Autodesk Inventor part; units mm, degrees
ref_plane "YZ Plane" through (0, 0, 0) normal (1, 0, 0) x (0, 1, 0)
ref_plane "XZ Plane" through (0, 0, 0) normal (0, 1, 0) x (-1, 0, 0)
ref_plane "XY Plane" through (0, 0, 0) normal (0, 0, 1) x (1, 0, 0)
sketch "Sketch1" plane through (0, 0, 0) normal (0, 0, 1) x (1, 0, 0)
  line L0 (-15, -15) -> (15, -15)
  line L1 (15, -15) -> (15, 15)
  line L2 (15, 15) -> (-15, 15)
  line L3 (-15, 15) -> (-15, -15)
  line L4 (-15, -15) -> (15, 15) construction
  line L5 (15, -15) -> (-15, 15) construction
  point P0 (0, 0)
  dimension "d0" = 30
  dimension "d1" = 30
extrude "Extrusion1" add sketch "Sketch1" along normal blind 4.7
sketch "Sketch2" plane through (0, 0, 4.7) normal (0, 0, 1) x (1, 0, 0)
  point P0 (0, 0)
hole "Hole1" at (0, 0, 4.7) direction (0, 0, -1) diameter 21 end through all
sketch "Sketch3" plane through (0, 0, 0) normal (0, 1, 0) x (-1, 0, 0)
  line L0 (-10.5, 6.7) -> (-13, 6.7)
  line L1 (-13, 6.7) -> (-13, 4.7)
  line L2 (-13, 4.7) -> (-10.5, 4.7)
  line L3 (-10.5, 4.7) -> (-10.5, 6.7)
  line L4 (-15, 4.7) -> (15, 4.7)
  line L5 (-10.5, 0) -> (-10.5, 4.7)
  line L6 (0, 0) -> (0, 4.7)
  line L7 (10.5, 0) -> (-10.5, 0)
  dimension "d13" = 26
  dimension "d15" = 2
revolve "Revolution1" add sketch "Sketch3" angle 360 about axis through (0, 0, 0) along (0, 0, 1) contours L3 L2 L1 L0
sketch "Sketch4" plane through (0, 0, 0) normal (0, 0, -1) x (-1, 0, 0)
  line L0 (-11, -11) -> (11, -11)
  line L1 (11, -11) -> (11, 11)
  line L2 (11, 11) -> (-11, 11)
  line L3 (-11, 11) -> (-11, -11)
  line L4 (-11, -11) -> (11, 11) construction
  line L5 (11, -11) -> (-11, 11) construction
  point P0 (0, 0)
  point P1 (0, 0)
  dimension "d17" = 22
hole "Hole2" at (11, 11, 0) at (-11, 11, 0) at (-11, -11, 0) at (11, -11, 0) direction (0, 0, 1) diameter 3.4 end through all counterbore diameter 6.5 counterbore depth 3.4
chamfer "Chamfer1" distance 2 angle 45 4 edges at (15, -15, 2.35) (15, 15, 2.35) (-15, 15, 2.35) (-15, -15, 2.35)
chamfer "Chamfer2" distance 0.7 angle 45 1 edges at (0, 10.5, 0)
properties part number "Festlager Deckel" material "Aluminum 6061"
For this review, take the finished solid that the model builds, in its own axes (mm). A direction names the side the tool comes from. Coordinates: 2 decimals unless noted, no trailing zeros. Loops run counter-clockwise (first coordinate to the right, second up) from the corner with the lowest first, then second, coordinate; pieces in that order, holes last. Notation, with made-up numbers: (-23, 67) -> (33, 67) arc R17 ccw to (33, 96) -> close; hole circle Ø3 at (-18.5, 44). An arc over 180 degrees is marked (long way). Return JSON: item names as keys, results as strings. Group by question number.
(1) Consider section A-A, the plane x = 0. Give the boundary of the cut face in (y, z).
(2) Consider section D-D, the plane z = 6. Give the boundary of the cut face in (x, y).
(3) To check wall thickness, follow L1, parallel to X at y = -11, z = 3.25; L2, parallel to X at y = -11, z = 3.75. State the ranges of each line that lie inside material, in increasing order.
(4) Consider section B-B, the plane z = 4. Give the boundary of the cut face in (x, y).
(5) Mouldability with a two-part tool opening along X and no side actions: class faces 1 (the flat face through (12.4, 12.4, 3.4)), 2 (the flat face through (13, -3, 4.7)), 3 (the flat face through (-14, -14, 2)) as pulls with the +X half, pulls with the -X half, needs draft (parallel to the pull), parting line crosses it, or undercut.
(6) Consider section C-C, the plane y = -11.75. Give the boundary of the cut face in (x, z).
(7) For pin 1 Ø5.5 at (x, y) = (11, 11) entering from +Z; pin 2 Ø4 at (x, y) = (11, -11) entering from -Z; pin 3 Ø4 at (x, y) = (11, -11) entering from +Z; pin 4 Ø6 at (x, y) = (-0.5, -8) entering from -Z, all flat-tipped, find the tip position at first contact; note any pin that passes through.
(8) Tool access review of faces 4 (the cylindrical face through (-10.316, 7.91, 5.686)), 5 (the cylindrical face through (10.857, 7.753, 1.724)), 6 (the flat face through (-15, 0, 2)): name each direction out of +Z, -Z, +X, -X, +Y, -Y from which nothing blocks a thin tool from reaching the whole face with its end or side.
Results below:
{
 "1": {"outline": "(-15, 0) -> (-11.2, 0) -> (-10.5, 0.7) -> (-10.5, 6.7) -> (-13, 6.7) -> (-13, 4.7) -> (-15, 4.7) -> close; (10.5, 0.7) -> (11.2, 0) -> (15, 0) -> (15, 4.7) -> (13, 4.7) -> (13, 6.7) -> (10.5, 6.7) -> close"},
 "2": {"outline": "circle Ø26 at (0, 0); hole circle Ø21 at (0, 0)"},
 "3": {"L1": "x = -15 to -14.25, -7.75 to 7.75, 14.25 to 15", "L2": "x = -15 to -12.7, -9.3 to 9.3, 12.7 to 15"},
 "4": {"outline": "(-15, -13) -> (-13, -15) -> (13, -15) -> (15, -13) -> (15, 13) -> (13, 15) -> (-13, 15) -> (-15, 13) -> close; hole circle Ø3.4 at (-11, -11); hole circle Ø3.4 at (-11, 11); hole circle Ø21 at (0, 0); hole circle Ø3.4 at (11, -11); hole circle Ø3.4 at (11, 11)"},
 "5": {"face 1": "undercut", "face 2": "needs draft", "face 3": "pulls with the -X half"},
 "6": {"outline": "(-15, 0) -> (-14.16, 0) -> (-14.16, 3.4) -> (-12.53, 3.4) -> (-12.53, 4.7) -> (-15, 4.7) -> close; (-9.47, 3.4) -> (-7.84, 3.4) -> (-7.84, 0) -> (7.84, 0) -> (7.84, 3.4) -> (9.47, 3.4) -> (9.47, 4.7) -> (5.56, 4.7) -> (5.56, 6.7) -> (-5.56, 6.7) -> (-5.56, 4.7) -> (-9.47, 4.7) -> close; (12.53, 3.4) -> (14.16, 3.4) -> (14.16, 0) -> (15, 0) -> (15, 4.7) -> (12.53, 4.7) -> close"},
 "7": {"pin 1": "stops at z = 6.7", "pin 2": "stops at z = 3.4", "pin 3": "stops at z = 4.7", "pin 4": "stops at z = 0.18"},
 "8": {"face 4": "+Z", "face 5": "-Z", "face 6": "+Z, -Z, -X, +Y, -Y"}
}
